Geometry check sheet. Reference: the model listing, model coordinates, mm. A direction names the side the tool comes from. Round coordinates to 2 decimals unless told otherwise and drop trailing zeros. Loops run counter-clockwise (first coordinate to the right, second up) from the corner with the lowest first, then second, coordinate; pieces in that order, holes last. Notation, with made-up numbers: (65.5, -14.75) -> (73.5, -14.75) arc R14 ccw to (73.5, -8.75) -> close; hole circle Ø6 at (29, 9). An arc over 180 degrees is marked (long way). Use a Markdown table: item, result. Add a question column.
Q1. Sectioned sample at D-D, the plane z = 2. Enter the section's corners in (x, y), then the cut area to 3 significant figures.
Q2. Gauge pin test, flat ends, axial feed: P1, Ø1, axis at y = 12.5, z = 4, coming from the +X side; P2, Ø5, axis at x = 5, y = 19.5, coming from the -Z side; P3, Ø5.5, axis at y = 30.5, z = 3, coming from the +X side; P4, Ø5, axis at x = -4.5, z = 6.5, coming from the +Y side. Record the tip position at first contact, or that the pin passes through.
Q3. Set-up check for faces 1 (the face through (6.5, 32, 0)), 2 (the face through (9, 31, 6.75)), 3 (the face through (0, 25, 0)), 4 (the face through (20, 27, 0)): record each of +Z, -Z, +X, -X, +Y, -Y from which the full face is reachable in a straight line by a thin tool's end or side.
Q4. Sectioned sample at C-C, the plane y = 23.5. Enter the section's corners in (x, z), then the cut area to 3 significant figures.
Q5. Sectioned sample at B-B, the plane x = 7. Enter the section's corners in (y, z), then the cut area to 3 significant figures.
Q6. Sectioned sample at A-A, the plane z = 0. Enter the section's corners in (x, y).
Q7. Material ranges on L1, parallel to Z at x = 0, y = 17; L2, parallel to Y at x = 7.5, z = -2, recorded low to high.
Q8. Release check for a two-part mould opening along X. For faces 5 (the face through (9, 31, -6.75)), 6 (the face through (21, 27, -3)), 7 (the face through (25, 27, 0)), 8 (the face through (23, 27, 0)) record: released by +X, released by -X, zero draft, split by the parting line, or undercut.
```python
from build123d import *

# Parameters (mm, degrees)
SKETCH1_R           = 10
SKETCH1_R_2         = 6.5
BOSS_EXTRUDE1_DEPTH = 25
BOSS_EXTRUDE2_DEPTH = 4
SKETCH3_W           = 6
SKETCH3_H           = 13.5
BOSS_EXTRUDE3_DEPTH = 5
SKETCH4_W           = 7
SKETCH4_H           = 2
CUT_EXTRUDE1_DEPTH  = 12
SKETCH5_W           = 3
SKETCH5_H           = 6
CUT_EXTRUDE2_DEPTH  = 12


with BuildPart() as part:
    # Sketch1 → Boss-Extrude1 (new body)
    with BuildSketch(Plane(origin=(0, 0, 0), x_dir=(1, 0, 0), z_dir=(0, 1, 0))):
        Circle(SKETCH1_R)
        Circle(SKETCH1_R_2, mode=Mode.SUBTRACT)
    extrude(amount=BOSS_EXTRUDE1_DEPTH)

    # Sketch2 → Boss-Extrude2 (add)
    with BuildSketch(Plane(origin=(0, 25, 0), x_dir=(1, 0, 0), z_dir=(0, 1, 0))):
        with BuildLine():
            Line((0, 10), (25, 10))
            Line((25, 10), (25, -10))
            Line((25, -10), (0, -10))
            ThreePointArc((0, -10), (-10, 0), (0, 10))
        make_face()
    extrude(amount=BOSS_EXTRUDE2_DEPTH)

    # Sketch3 → Boss-Extrude3 (add)
    with BuildSketch(Plane(origin=(0, 29, 0), x_dir=(1, 0, 0), z_dir=(0, 1, 0))):
        with Locations((9.5, 0)):
            Rectangle(SKETCH3_W, SKETCH3_H)
    extrude(amount=BOSS_EXTRUDE3_DEPTH)

    # Sketch4 → Cut-Extrude1 (cut)
    with BuildSketch(Plane(origin=(12.5, 0, 0), x_dir=(0, 0, -1), z_dir=(1, 0, 0))):
        with Locations((0, 30)):
            Rectangle(SKETCH4_W, SKETCH4_H)
    extrude(amount=-CUT_EXTRUDE1_DEPTH, mode=Mode.SUBTRACT)

    # Sketch5 → Cut-Extrude2 (cut)
    with BuildSketch(Plane(origin=(0, 29, 0), x_dir=(1, 0, 0), z_dir=(0, 1, 0))):
        with Locations((21.5, 0)):
            Rectangle(SKETCH5_W, SKETCH5_H)
    extrude(amount=-CUT_EXTRUDE2_DEPTH, mode=Mode.SUBTRACT)


solid = part.part
```
Values:
| question | item | result |
|---|---|---|
| 1 | outline | (-9.8, 0) -> (-6.18, 0) -> (-6.18, 25) -> (6.18, 25) -> (6.18, 0) -> (9.8, 0) -> (9.8, 25) -> (20, 25) -> (20, 29) -> (-9.8, 29) -> close; (6.5, 31) -> (12.5, 31) -> (12.5, 34) -> (6.5, 34) -> close; (23, 25) -> (25, 25) -> (25, 29) -> (23, 29) -> close |
| 1 | area | 326 mm^2 |
| 2 | P1 | x = 9.37 |
| 2 | P2 | z = -9.68 |
| 2 | P3 | x = 25 |
| 2 | P4 | y = 29 |
| 3 | face 1 | +Z, -Z, -X, +Y |
| 3 | face 2 | +Z, +X, -X, +Y |
| 3 | face 3 | -Y |
| 3 | face 4 | +Y, -Y |
| 4 | outline | circle Ø20 at (0, 0); hole circle Ø13 at (0, 0) |
| 4 | area | 181 mm^2 |
| 5 | outline | (0, -7.14) -> (25, -7.14) -> (25, -10) -> (29, -10) -> (29, -6.75) -> (34, -6.75) -> (34, 6.75) -> (29, 6.75) -> (29, 10) -> (25, 10) -> (25, 7.14) -> (0, 7.14) -> close; hole (29, -3.5) -> (31, -3.5) -> (31, 3.5) -> (29, 3.5) -> close |
| 5 | area | 491 mm^2 |
| 6 | outline | (-10, 0) -> (-6.5, 0) -> (-6.5, 25) -> (6.5, 25) -> (6.5, 0) -> (10, 0) -> (10, 25) -> (20, 25) -> (20, 29) -> (-10, 29) -> close; (6.5, 31) -> (12.5, 31) -> (12.5, 34) -> (6.5, 34) -> close; (23, 25) -> (25, 25) -> (25, 29) -> (23, 29) -> close |
| 7 | L1 | -10 to -6.5, 6.5 to 10 |
| 7 | L2 | 0 to 29, 31 to 34 |
| 8 | face 5 | zero draft |
| 8 | face 6 | undercut |
| 8 | face 7 | released by +X |
| 8 | face 8 | undercut |
